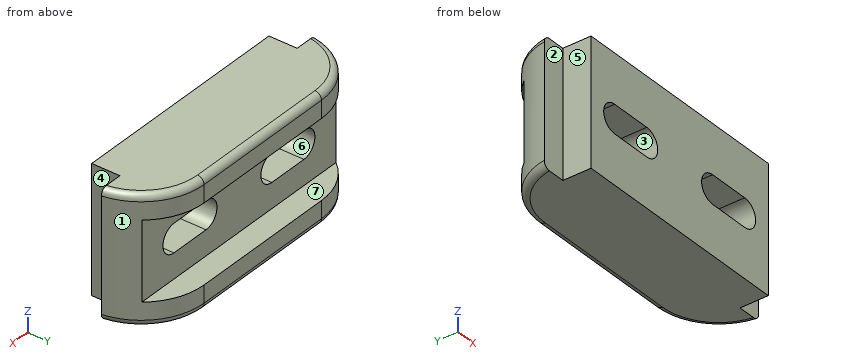
```python
from build123d import *

# Parameters (mm, degrees)
ESQUISSE1_W             = 127
ESQUISSE1_H             = 38
BASE_EXTRUSION_DEPTH    = 29
ESQUISSE2_W             = 11
ESQUISSE2_H             = 13
ENL_V_MAT_EXTRU_1_DEPTH = 95.022603665
CONG_1_R                = 29
ESQUISSE3_W             = 127
ESQUISSE3_H             = 36
ENL_V_MAT_EXTRU_2_DEPTH = 11
ENL_V_MAT_EXTRU_3_DEPTH = 75.848179671
CONG_2_R                = 3


with BuildPart() as part:
    # Esquisse1 → Base-Extrusion (new, symmetric)
    with BuildSketch(Plane.XY):
        with Locations((0, 19)):
            Rectangle(ESQUISSE1_W, ESQUISSE1_H)
    extrude(amount=BASE_EXTRUSION_DEPTH, both=True)

    # Esquisse2 → Enlèv. mat.-Extru.1 (cut, through all)
    with BuildSketch(Plane.XY.offset(29)):
        with Locations((-58, 6.5)):
            Rectangle(ESQUISSE2_W, ESQUISSE2_H)
        with Locations((58, 6.5)):
            Rectangle(ESQUISSE2_W, ESQUISSE2_H)
    extrude(amount=-ENL_V_MAT_EXTRU_1_DEPTH, mode=Mode.SUBTRACT)

    # Congé1
    # the kernel refuses this fillet: 29 mm, written as the material it takes off along each edge
    with BuildSketch(Plane(origin=(-63.5, 38, 100.807033082), x_dir=(0, -1, 0), z_dir=(0, 0, -1))) as cong_1_piece_1:
        with BuildLine():
            CenterArc((29, -28.722813233), CONG_1_R, 97.928141766, 82.071858234)
            Line((0, -28.722813233), (-0.58, -28.722813233))
            Line((-0.58, -28.722813233), (-0.58, 0))
            Line((-0.58, 0), (0, 0.58))
            ThreePointArc((0, 0.58), (12.5, 0.58), (24.92, 0.574456265))
            Line((24.92, 0.574456265), (25, 0))
        make_face()
    extrude(amount=201.614066163, mode=Mode.SUBTRACT)
    with BuildSketch(Plane(origin=(63.5, 38, -100.807033082), x_dir=(-1, 0, 0), z_dir=(0, 0, 1))) as cong_1_piece_2:
        with BuildLine():
            CenterArc((28.722813233, 29), CONG_1_R, 187.928141766, 82.071858234)
            Line((0, 25), (-0.574456265, 24.92))
            ThreePointArc((-0.574456265, 24.92), (-0.58, 12.5), (-0.58, 0))
            Line((-0.58, 0), (0, -0.58))
            Line((0, -0.58), (28.722813233, -0.58))
            Line((28.722813233, -0.58), (28.722813233, 0))
        make_face()
    extrude(amount=201.614066163, mode=Mode.SUBTRACT)

    # Esquisse3 → Enlèv. mat.-Extru.2 (cut)
    with BuildSketch(Plane(origin=(0, 38, 0), x_dir=(-1, 0, 0), z_dir=(0, 1, 0))):
        Rectangle(ESQUISSE3_W, ESQUISSE3_H)
    extrude(amount=-ENL_V_MAT_EXTRU_2_DEPTH, mode=Mode.SUBTRACT)

    # Esquisse4 → Enlèv. mat.-Extru.3 (cut, through all)
    with BuildSketch(Plane(origin=(0, 27, 0), x_dir=(-1, 0, 0), z_dir=(0, 1, 0))):
        with BuildLine():
            Line((19.5, -6.5), (38.5, -6.5))
            ThreePointArc((38.5, -6.5), (45, 0), (38.5, 6.5))
            Line((38.5, 6.5), (19.5, 6.5))
            ThreePointArc((19.5, 6.5), (13, 0), (19.5, -6.5))
        make_face()
    enl_v_mat_extru_3 = extrude(amount=-ENL_V_MAT_EXTRU_3_DEPTH, mode=Mode.SUBTRACT)

    # Symétrie1: Enlèv. mat.-Extru.3 across plane
    add(enl_v_mat_extru_3.mirror(Plane(origin=(0, 0, 0), x_dir=(0, 0, 1), z_dir=(1, 0, 0))), mode=Mode.SUBTRACT)

    # Congé2
    cong_2_edges = [part.edges().sort_by_distance(p)[0] for p in [
        (0, 38, -29),
        (53.816619532, 30.874642854, -29),
        (-53.816619532, 30.874642854, -29),
        (0, 38, 29),
        (53.816619532, 30.874642854, 29),
        (-53.816619532, 30.874642854, 29),
    ]]
    fillet(cong_2_edges, radius=CONG_2_R)


solid = part.part
```
Model file for the job. Use its own axes, mm. Face numbers are marked on the shaded views. A direction names the side the tool comes from. Give positions to 0.01 mm unless a question says otherwise; leave off trailing zeros. Order: outer loops, then holes, each group sorted by start corner. A loop starts at its lowest first (then second) coordinate and runs counter-clockwise, first axis right, second up.
1) Pin check, flat tips, straight feed: pin 1 (12 mm diameter, centred on x = 57.5, z = 9.5, fed in from -Y); pin 2 (10.5 mm diameter, centred on y = 8.5, z = 12, fed in from +X); pin 3 (5 mm diameter, centred on x = 36, z = 13, fed in from +Y); pin 4 (5.5 mm diameter, centred on x = -57, z = -7.5, fed in from -Y). Stop position of each tip, or through.
2) Saw through at D-D, the plane z = -13.5. Write the cut outline in (x, y).
3) 3-axis set-ups, long thin cutter, end or side, ignore diameter. For the marked faces 4, 5, 6 and 7: which of +Z, -Z, +X, -X, +Y, -Y reach the whole face in a straight line?
4) Saw through at A-A, the plane x = 21. Write the cut outline in (y, z), then the cut area to 3 significant figures.
5) Saw through at B-B, the plane y = 11. Write the cut outline in (x, z), then the cut area to 3 significant figures.
6) Wall check: probe 1 along Z at (x, y) = (-31, 17); probe 2 along Z at (x, y) = (12.5, 30.5); probe 3 along X at (y, z) = (9.5, 2). Give the ranges that are in metal, low to high.
7) Mould opens along X. For the marked faces 1, 2 and 3 say: +X half, -X half, draft (parallel to the pull), parting line (faces both ways), or undercut.
8) Saw through at C-C, the plane z = 20. Write the cut outline in (x, y).
Computed:
1. pin 1: stops at y = 0
1. pin 2: stops at x = 63.5
1. pin 3: stops at y = 27
1. pin 4: stops at y = 13
2. outline: (-63.5, 13) - (-52.5, 13) - (-52.5, 0) - (52.5, 0) - (52.5, 13) - (63.5, 13) arc R29 ccw to (57.51, 27) - (-57.51, 27) arc R29 ccw to start
3. face 4: +Z, -Z, +X, -Y
3. face 5: +Z, -Z, -X, -Y
3. face 6: +Y, -Y
3. face 7: +X, -X, +Y
4. outline: (0, -29) - (35, -29) arc R3 ccw to (38, -26) - (38, -18) - (27, -18) - (27, -6.5) - (0, -6.5) - close; (0, 6.5) - (27, 6.5) - (27, 18) - (38, 18) - (38, 26) arc R3 ccw to (35, 29) - (0, 29) - close
4. area: 1,450 mm2
5. outline: (-52.5, -29) - (52.5, -29) - (52.5, 29) - (-52.5, 29) - close; hole (-38.5, -6.5) - (-19.5, -6.5) arc R6.5 ccw to (-19.5, 6.5) - (-38.5, 6.5) arc R6.5 ccw to start; hole (19.5, -6.5) - (38.5, -6.5) arc R6.5 ccw to (38.5, 6.5) - (19.5, 6.5) arc R6.5 ccw to start
5. area: 5,330 mm2
6. probe 1: z = -29 to -6.5, 6.5 to 29
6. probe 2: z = -29 to -18, 18 to 29
6. probe 3: x = -52.5 to -44.68, -13.32 to 13.32, 44.68 to 52.5
7. face 1: +X half
7. face 2: draft
7. face 3: undercut
8. outline: (-63.5, 13) - (-52.5, 13) - (-52.5, 0) - (52.5, 0) - (52.5, 13) - (63.5, 13) arc R29 ccw to (34.78, 38) - (-34.78, 38) arc R29 ccw to start
